from build123d import *

# Parameters (mm, degrees)
SKETCH1_R               = 25.4
BOSS_EXTRUDE1_DEPTH     = 2.794
SKETCH2_R               = 4.7625
SKETCH2_R_2             = 1.27
CUT_EXTRUDE1_DEPTH      = 37.353070627
CUT_EXTRUDE2_START      = -1.27
SKETCH3_R               = 22.86
CUT_EXTRUDE2_DEPTH      = 1.651
CUT_EXTRUDE3_DEPTH      = 37.029521729
CUT_EXTRUDE3_DEPTH_BACK = 37.029521729
SKETCH4_R               = 4.7625


with BuildPart() as part:
    # Sketch1 → Boss-Extrude1 (new, symmetric)
    with BuildSketch(Plane.XY):
        Circle(SKETCH1_R)
    extrude(amount=BOSS_EXTRUDE1_DEPTH, both=True)

    # Sketch2 → Cut-Extrude1 (cut, through all)
    with BuildSketch(Plane.XY.offset(2.794)):
        Circle(SKETCH2_R)
        with Locations((0, 7.9375)):
            Circle(SKETCH2_R_2)
        with Locations((5.612952969, 5.613367182)):
            Circle(SKETCH2_R_2)
        with Locations((7.9385, 0.001)):
            Circle(SKETCH2_R_2)
        with Locations((5.614367182, -5.611952969)):
            Circle(SKETCH2_R_2)
        with Locations((0.002, -7.9375)):
            Circle(SKETCH2_R_2)
        with Locations((-5.610952969, -5.613367182)):
            Circle(SKETCH2_R_2)
        with Locations((-7.9365, -0.001)):
            Circle(SKETCH2_R_2)
        with Locations((-5.612367182, 5.611952969)):
            Circle(SKETCH2_R_2)
    extrude(amount=-CUT_EXTRUDE1_DEPTH, mode=Mode.SUBTRACT)

    # Sketch3 → Cut-Extrude2 (cut)
    with BuildSketch(Plane.XY.offset(CUT_EXTRUDE2_START)):
        Circle(SKETCH3_R)
    cut_extrude2 = extrude(amount=-CUT_EXTRUDE2_DEPTH, mode=Mode.SUBTRACT)

    # Mirror1: Cut-Extrude2 across plane
    add(cut_extrude2.mirror(Plane.XY), mode=Mode.SUBTRACT)

    # Sketch4 → Cut-Extrude3 (cut, two sides: drawn at the far end of the back side and taken through both)
    with BuildSketch(Plane.XY.offset(-CUT_EXTRUDE3_DEPTH_BACK)):
        with Locations((0, 17.4625)):
            Circle(SKETCH4_R)
        with Locations((12.347852166, 12.347852166)):
            Circle(SKETCH4_R)
        with Locations((17.4625, 0)):
            Circle(SKETCH4_R)
        with Locations((12.347852166, -12.347852166)):
            Circle(SKETCH4_R)
        with Locations((0, -17.4625)):
            Circle(SKETCH4_R)
        with Locations((-12.347852166, -12.347852166)):
            Circle(SKETCH4_R)
        with Locations((-17.4625, 0)):
            Circle(SKETCH4_R)
        with Locations((-12.347852166, 12.347852166)):
            Circle(SKETCH4_R)
    extrude(amount=CUT_EXTRUDE3_DEPTH + CUT_EXTRUDE3_DEPTH_BACK, mode=Mode.SUBTRACT)


solid = part.part
Model file for the job. Use its own axes, mm. A direction names the side the tool comes from. Give positions to 0.01 mm unless a question says otherwise; leave off trailing zeros. Order: outer loops, then holes, each group sorted by start corner. A loop starts at its lowest first (then second) coordinate and runs counter-clockwise, first axis right, second up. Notation, with made-up numbers: M 56.5,56.5 L 113.5,56.5 A22 cw 113.5,62.5 Z; hole C 33.5,66.5 d11. An arc over 180 degrees is marked long. Put each result on its own line as item: value. Start each with the question number.
(1) Band-saw the part on A-A on x = 0. Count the separate pieces of the cut face and the enclosed holes in it, then the cut area to 3 significant figures.
(2) Band-saw the part on C-C on x = 10. Give the cut face in (y, z).
(3) Tool access for faces 4 (the face through (0, -5, -1.27)), 5 (the face through (21.804, 6.867, 2.021)), 6 (the face through (7.59, -12.14, -0.02)): list every direction of +Z, -Z, +X, -X, +Y, -Y with a clear straight run to the whole face (end or side of a thin tool).
(4) Pull direction Y, two halves, no side cores. Call faces 1 (the face through (-22.22, 0.21, -0.02)), 2 (the face through (-21, 10, 2.794)), 3 (the face through (-5.506, -24.796, 0.039)): released by +Y, released by -Y, zero draft, split by the parting line, or undercut.
(5) Band-saw the part on B-B on y = -18.5. Give the cut face in (x, z), then the cut area to 3 significant figures.
(6) Drill centre lines: L1, parallel to Y at x = -15, z = 0.55; L2, parallel to Y at x = 2, z = 0.65; L3, parallel to X at y = -9.5, z = -0.3. Where is each one in solid material? Low to high. Write a range as [from, to].
(7) Band-saw the part on D-D on z = 2. Give the cut face in (x, y), then the cut area to 3 significant figures.
(8) Pin check, flat tips, straight feed: pin 1 Ø12.5 at (x, y) = (17.46, 0) entering from +Z; pin 2 Ø2 at (x, y) = (-9.5, -15) entering from -Z; pin 3 Ø7.5 at (x, y) = (12.35, 12.35) entering from +Z; pin 4 Ø1 at (y, z) = (-19, 2) entering from +X. Stop position of each tip, or through.
Results below:
1. separate pieces: 6
1. enclosed holes: 0
1. area: 59.0 mm2
2. outline: M -23.35,-2.79 L -20.56,-2.79 L -20.56,-1.27 L -16.49,-1.27 L -16.49,1.27 L -20.56,1.27 L -20.56,2.79 L -23.35,2.79 Z; M -8.2,-1.27 L 8.2,-1.27 L 8.2,1.27 L -8.2,1.27 Z; M 16.49,-1.27 L 20.56,-1.27 L 20.56,-2.79 L 23.35,-2.79 L 23.35,2.79 L 20.56,2.79 L 20.56,1.27 L 16.49,1.27 Z
3. face 4: -Z
3. face 5: +Z
3. face 6: +Z, -Z
4. face 1: undercut
4. face 2: zero draft
4. face 3: split by the parting line
5. outline: M -17.4,-2.79 L -13.43,-2.79 L -13.43,-1.27 L -4.65,-1.27 L -4.65,1.27 L -13.43,1.27 L -13.43,2.79 L -17.4,2.79 Z; M 4.65,-1.27 L 13.43,-1.27 L 13.43,-2.79 L 17.4,-2.79 L 17.4,2.79 L 13.43,2.79 L 13.43,1.27 L 4.65,1.27 Z
5. area: 89.0 mm2
6. L1: y = [-20.5, -16.3], [-8.39, -4.08], [4.08, 8.39], [16.3, 20.5]
6. L2: y = [-25.32, -21.78], [-13.14, -4.32], [4.32, 13.14], [21.78, 25.32]
6. L3: x = [-23.56, -16.17], [-8.53, 8.53], [16.17, 23.56]
7. outline: C 0,0 d50.8; hole C 0,0 d45.72
7. area: 385 mm2
8. pin 1: stops at z = 2.79
8. pin 2: stops at z = -1.27
8. pin 3: passes through
8. pin 4: stops at x = 17.4
